The figure shows three views and two pictorial views of one solid part (mm, origin at its lowest corner). Answer the questions. Coordinates: 2 decimals unless noted, no trailing zeros. Order: outer loops, then holes, each group sorted by start corner. A loop starts at its lowest first (then second) coordinate and runs counter-clockwise, first axis right, second up. Notation, with made-up numbers: (73.5, 50) -> (100.5, 50) arc R28 ccw to (100.5, 88) -> close; hole circle Ø7 at (86.5, -7.75). An arc over 180 degrees is marked (long way). Return JSON: item names as keys, results as strings.
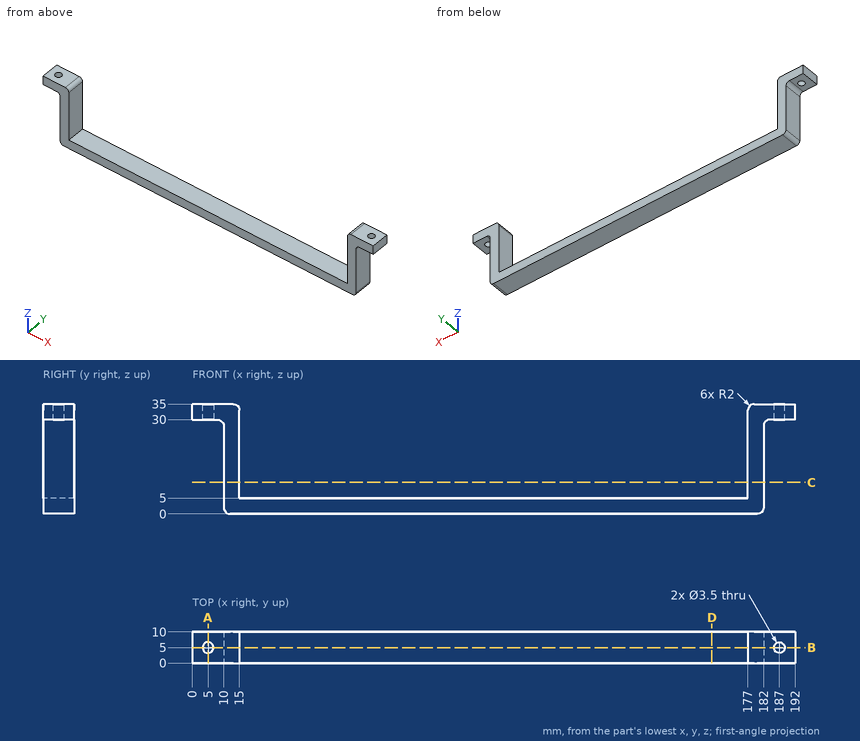
1. The part is cut by section D-D on x = 165.5. Give the vertices of the cut face in (y, z).
Answer block:
{"outline": "(0, 0) -> (10, 0) -> (10, 5) -> (0, 5) -> close"}
2. The part is cut by section B-B on y = 5. Give the vertices of the cut face in (x, z).
Answer block:
{"outline": "(0, 30) -> (3.25, 30) -> (3.25, 35) -> (0, 35) -> close; (6.75, 30) -> (8, 30) arc R2 cw to (10, 28) -> (10, 2) arc R2 ccw to (12, 0) -> (180, 0) arc R2 ccw to (182, 2) -> (182, 28) arc R2 cw to (184, 30) -> (185.25, 30) -> (185.25, 35) -> (179, 35) arc R2 ccw to (177, 33) -> (177, 5) -> (15, 5) -> (15, 33) arc R2 ccw to (13, 35) -> (6.75, 35) -> close; (188.75, 30) -> (192, 30) -> (192, 35) -> (188.75, 35) -> close"}
3. Consider line 1 (X direction, y = 1.75, z = 20); line 2 (X direction, y = 5.75, z = 31); line 3 (Y direction, x = 187, z = 33.9). Determine where each line is inside the solid, lowest interval first. Write a range as from..to.
Answer block:
{"line 1": "x = 10..15, 177..182", "line 2": "x = 0..3.42, 6.58..15, 177..185.42, 188.58..192", "line 3": "y = 0..3.25, 6.75..10"}
4. The part is cut by section A-A on x = 5. Give the vertices of the cut face in (y, z).
Answer block:
{"outline": "(0, 30) -> (3.25, 30) -> (3.25, 35) -> (0, 35) -> close; (6.75, 30) -> (10, 30) -> (10, 35) -> (6.75, 35) -> close"}
5. The part is cut by section C-C on z = 10. Give the vertices of the cut face in (x, y), and give its area (3 significant figures).
Answer block:
{"outline": "(10, 0) -> (15, 0) -> (15, 10) -> (10, 10) -> close; (177, 0) -> (182, 0) -> (182, 10) -> (177, 10) -> close", "area": "100 mm2"}
6. Each of these flat-tipped pins is pushed along its axis until it touches: pin 1 Ø5 at (y, z) = (6.5, 24.5) entering from +X; pin 2 Ø5 at (x, y) = (134.5, 8) entering from +Z; pin 3 Ø4 at (x, y) = (2.5, 4.5) entering from -Z; pin 4 Ø12 at (x, z) = (163, 13.5) entering from -Y. Where does it stop, or does it pass through?
Answer block:
{"pin 1": "stops at x = 182", "pin 2": "stops at z = 5", "pin 3": "stops at z = 30", "pin 4": "passes through"}
